Geometry: final body of the model. Coordinates: model frame, mm. A direction names the side the tool comes from. Give positions to 0.01 mm unless a question says otherwise; leave off trailing zeros. Loops run counter-clockwise (first coordinate to the right, second up) from the corner with the lowest first, then second, coordinate; pieces in that order, holes last.
Solid Edge part; units mm, degrees
sketch "Sketch1" plane through (0, 0, 0) normal (0, -1, 0) x (1, 0, 0)
  line L0 (-7.5, -5) -> (7.5, -5)
  line L1 (7.5, -5) -> (7.5, 5)
  line L2 (7.5, 5) -> (-7.5, 5)
  line L3 (-7.5, 5) -> (-7.5, -5)
  dimension "D1" = 7.5
  dimension "D2" = 7.5
extrude "Protrusion1" add sketch "Sketch1" along normal mid plane 72
sketch "Sketch2" plane through (0, 0, 5) normal (0, 0, 1) x (0, 1, 0)
  circle A0 centre (30.25, -3) radius 1.65
  circle A1 centre (-31.25, -4) radius 1.65
  circle A2 centre (-31.25, 4) radius 1.65
  circle A3 centre (30.25, 3) radius 1.65
  dimension "D1" = 30.25
  dimension "D2" = 31.25
extrude "Cutout1" cut sketch "Sketch2" against normal through all
fillet "Redondeo_1" radius 5 2 edges at (7.5, 0, 5) (-7.5, 0, 5)
sketch "Sketch3" plane through (0, 0, 5) normal (0, 0, 1) x (0, 1, 0)
  circle A0 centre (-31.25, 4) radius 3
  circle A1 centre (30.25, 3) radius 3.01
  circle A2 centre (-31.25, -4) radius 3
  circle A3 centre (30.25, -3) radius 3.01
extrude "VaciadoExtruido_3" cut sketch "Sketch3" against normal blind 4
fillet "Redondeo_2" radius 2 10 edges at (-7.5, 36, -2.5) (-6.0355, 36, 3.5355) (0, 36, 5) (6.0355, 36, 3.5355) (7.5, 36, -2.5) (0, -36, 5) (-6.0355, -36, 3.5355) (-7.5, -36, -2.5) (6.0355, -36, 3.5355) (7.5, -36, -2.5)
Item 1: Draft query along X for faces 3 (the face through (-0.04, -35.43, 4.4)), 4 (the face through (-1.07, -31.9, 2.58)), 5 (the face through (-7.5, 0, -2)), 6 (the face through (6, 0.48, 3.57)). Return one class per face: +X half, -X half, draft (parallel to the pull), parting line (faces both ways), or undercut.
Values follow:
face 3: draft
face 4: undercut
face 5: -X half
face 6: +X half
Item 2: Pin query (flat end, axial travel): pin 1 (4 mm diameter, centred on x = -4, y = -31.25, fed in from +Z); pin 2 (2.5 mm diameter, centred on x = -3, y = 30.25, fed in from -Z); pin 3 (5 mm diameter, centred on x = 5, y = -32, fed in from +Z). Return the tip coordinate at first contact, or that it passes through.
Values follow:
pin 1: stops at z = 1
pin 2: passes through
pin 3: stops at z = 4.8
Item 3: Set-up query: faces 1 (the face through (-3, -33, 1)), 2 (the face through (0, -2, 5)). Return all of +Z, -Z, +X, -X, +Y, -Y with unobstructed straight access to the full face (end or side cutting, diameter ignored); none if empty.
Values follow:
face 1: +Z
face 2: +Z, +X, -X, +Y, -Y
Item 4: Section query C-C on y = 26.5. Return loops of the section in (x, z), plus the area to 3 significant figures.
Values follow:
outline: (-7.5, -5) - (7.5, -5) - (7.5, 0) arc R5 ccw to (2.5, 5) - (-2.5, 5) arc R5 ccw to (-7.5, 0) - close
area: 139 mm2
Item 5: Section query B-B on z = -3.25. Return loops of the section in (x, y).
Values follow:
outline: (-7.5, -34) arc R2 ccw to (-5.5, -36) - (5.5, -36) arc R2 ccw to (7.5, -34) - (7.5, 34) arc R2 ccw to (5.5, 36) - (-5.5, 36) arc R2 ccw to (-7.5, 34) - close; hole circle Ø3.3 at (-4, -31.25); hole circle Ø3.3 at (-3, 30.25); hole circle Ø3.3 at (3, 30.25); hole circle Ø3.3 at (4, -31.25)
Item 6: Ray query, probe 1 along X at (y, z) = (-31.25, -2.45); probe 2 along Y at (x, z) = (-4, -0.9); probe 3 along Y at (x, z) = (-0.75, 2.5). Return the intervals inside material, ascending.
Values follow:
probe 1: x = -7.5 to -5.65, -2.35 to 2.35, 5.65 to 7.5
probe 2: y = -36 to -32.9, -29.6 to 28.94, 31.56 to 36
probe 3: y = -36 to 28.25, 32.25 to 36
Item 7: Section query A-A on y = -31.25. Return loops of the section in (x, z), plus the area to 3 significant figures.
Values follow:
outline: (-7.5, -5) - (-5.65, -5) - (-5.65, 1) - (-7, 1) - (-7, 2.18) arc R5 ccw to (-7.5, 0) - close; (-2.35, -5) - (2.35, -5) - (2.35, 1) - (1, 1) - (1, 5) - (-1, 5) - (-1, 1) - (-2.35, 1) - close; (5.65, -5) - (7.5, -5) - (7.5, 0) arc R5 ccw to (7, 2.18) - (7, 1) - (5.65, 1) - close
area: 58.9 mm2
